Input: part model. Units: mm. Frame: model coordinates. Coordinates: 2 decimals unless noted, no trailing zeros. Order: outer loops, then holes, each group sorted by start corner. A loop starts at its lowest first (then second) coordinate and runs counter-clockwise, first axis right, second up. Notation, with made-up numbers: (-17.75, 18) -> (7.25, 18) arc R18 ccw to (7.25, 33) -> close; hole circle Ø9 at (52.25, 69). An arc over 180 degrees is marked (long way). Answer as CSV lines item,"result".
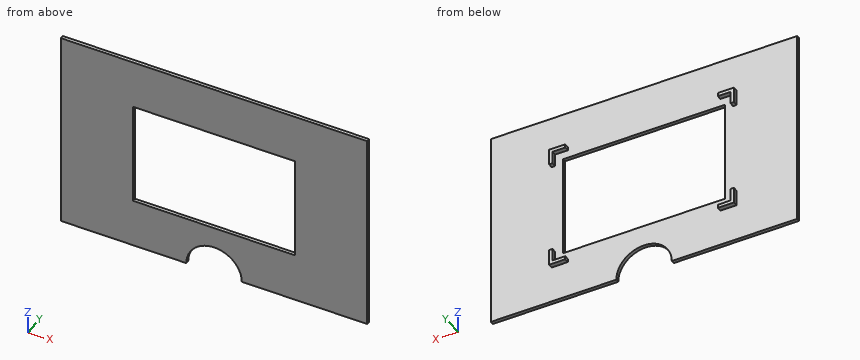
from build123d import *

# Parameters (mm, degrees)
SKETCH1_W           = 132.5
SKETCH1_H           = 87.5
BOSS_EXTRUDE1_DEPTH = 1.5
SKETCH2_W           = 80
SKETCH2_H           = 55
BOSS_EXTRUDE2_DEPTH = 2
SKETCH3_W           = 77
SKETCH3_H           = 52
CUT_EXTRUDE1_DEPTH  = 2
CUT_EXTRUDE2_REACH  = 3.5
SKETCH4_W           = 70
SKETCH4_H           = 45
SKETCH5_W           = 1.5
SKETCH5_H           = 41
SKETCH5_W_2         = 66
SKETCH5_H_2         = 1.5
CUT_EXTRUDE3_DEPTH  = 2
CUT_EXTRUDE4_DEPTH  = 1.5


with BuildPart() as part:
    # Sketch1 → Boss-Extrude1 (new body)
    with BuildSketch(Plane(origin=(0, 0, 0), x_dir=(1, 0, 0), z_dir=(0, 1, 0))):
        Rectangle(SKETCH1_W, SKETCH1_H)
    extrude(amount=BOSS_EXTRUDE1_DEPTH)

    # Sketch2 → Boss-Extrude2 (add)
    with BuildSketch(Plane(origin=(0, 1.5, 0), x_dir=(1, 0, 0), z_dir=(0, 1, 0))):
        Rectangle(SKETCH2_W, SKETCH2_H)
    extrude(amount=BOSS_EXTRUDE2_DEPTH)

    # Sketch3 → Cut-Extrude1 (cut)
    with BuildSketch(Plane(origin=(0, 3.5, 0), x_dir=(1, 0, 0), z_dir=(0, 1, 0))):
        Rectangle(SKETCH3_W, SKETCH3_H)
    extrude(amount=-CUT_EXTRUDE1_DEPTH, mode=Mode.SUBTRACT)

    # Sketch4 → Cut-Extrude2 (cut, up to next)
    with BuildSketch(Plane(origin=(0, 1.5, 0), x_dir=(1, 0, 0), z_dir=(0, 1, 0)), mode=Mode.PRIVATE) as cut_extrude2_sk1:
        Rectangle(SKETCH4_W, SKETCH4_H)
    cut_extrude2_tool1 = extrude(cut_extrude2_sk1.sketch, amount=-CUT_EXTRUDE2_REACH, mode=Mode.PRIVATE) & part.part
    add(cut_extrude2_tool1.solids().sort_by_distance((0, 1.5, 0))[0], mode=Mode.SUBTRACT)

    # Sketch5 → Cut-Extrude3 (cut)
    with BuildSketch(Plane(origin=(0, 3.5, 0), x_dir=(1, 0, 0), z_dir=(0, 1, 0))):
        with Locations((-39.25, 0)):
            Rectangle(SKETCH5_W, SKETCH5_H)
        with Locations((39.25, 0)):
            Rectangle(SKETCH5_W, SKETCH5_H)
        with Locations((0, 26.75)):
            Rectangle(SKETCH5_W_2, SKETCH5_H_2)
        with Locations((0, -26.75)):
            Rectangle(SKETCH5_W_2, SKETCH5_H_2)
    extrude(amount=-CUT_EXTRUDE3_DEPTH, mode=Mode.SUBTRACT)

    # Sketch6 → Cut-Extrude4 (cut)
    with BuildSketch(Plane(origin=(0, 1.5, 0), x_dir=(1, 0, 0), z_dir=(0, 1, 0))):
        with BuildLine():
            Line((-12, 43.75), (12, 43.75))
            ThreePointArc((12, 43.75), (0, 31.75), (-12, 43.75))
        make_face()
    extrude(amount=-CUT_EXTRUDE4_DEPTH, mode=Mode.SUBTRACT)


solid = part.part
1. Cut plane D-D (z = -24). Return the cut outline in (x, y).
Findings:
outline,"(-66.25, 0) -> (66.25, 0) -> (66.25, 1.5) -> (40, 1.5) -> (40, 3.5) -> (38.5, 3.5) -> (38.5, 1.5) -> (-38.5, 1.5) -> (-38.5, 3.5) -> (-40, 3.5) -> (-40, 1.5) -> (-66.25, 1.5) -> close"
2. Contact query for flat-ended pins moving along their axis: pin 1 (1.2 mm diameter, centred on y = 3, z = -27, fed in from +X); pin 2 (1.6 mm diameter, centred on y = 2.5, z = 24.5, fed in from -X); pin 3 (1.6 mm diameter, centred on x = 34.5, y = 3, fed in from +Z); pin 4 (12 mm diameter, centred on x = 22.5, z = 19, fed in from -Y). Output: stop coordinate, or through.
Findings:
pin 1,"stops at x = 40"
pin 2,"stops at x = -40"
pin 3,"stops at z = 27.5"
pin 4,"stops at y = 0"
3. Cut plane A-A (x = 0). Return the cut outline in (y, z), plus the area to 4 significant figures.
Findings:
outline,"(0, -31.75) -> (1.5, -31.75) -> (1.5, -22.5) -> (0, -22.5) -> close; (0, 22.5) -> (1.5, 22.5) -> (1.5, 43.75) -> (0, 43.75) -> close"
area,"45.75 mm2"
4. Cut plane B-B (y = 2.1). Return the cut outline in (x, z).
Findings:
outline,"(-40, -27.5) -> (-33, -27.5) -> (-33, -26) -> (-38.5, -26) -> (-38.5, -20.5) -> (-40, -20.5) -> close; (-40, 20.5) -> (-38.5, 20.5) -> (-38.5, 26) -> (-33, 26) -> (-33, 27.5) -> (-40, 27.5) -> close; (33, -27.5) -> (40, -27.5) -> (40, -20.5) -> (38.5, -20.5) -> (38.5, -26) -> (33, -26) -> close; (33, 26) -> (38.5, 26) -> (38.5, 20.5) -> (40, 20.5) -> (40, 27.5) -> (33, 27.5) -> close"
5. Cut plane C-C (z = 2). Return the cut outline in (x, y).
Findings:
outline,"(-66.25, 0) -> (-35, 0) -> (-35, 1.5) -> (-66.25, 1.5) -> close; (35, 0) -> (66.25, 0) -> (66.25, 1.5) -> (35, 1.5) -> close"
6. Ray query, line 1 along X through (y, z) = (0.9, 15.5); line 2 along Z through (x, y) = (28.5, 0.3); line 3 along X through (y, z) = (2.95, -26.5). Return the intervals inside material, ascending.
Findings:
line 1,"x = -66.25 to -35, 35 to 66.25"
line 2,"z = -43.75 to -22.5, 22.5 to 43.75"
line 3,"x = -40 to -33, 33 to 40"
